CAD build for the part. Positions are in the model's coordinates, mm. A direction names the side the tool comes from. Give positions to 0.01 mm unless a question says otherwise; leave off trailing zeros. Order: outer loops, then holes, each group sorted by start corner. A loop starts at its lowest first (then second) coordinate and runs counter-clockwise, first axis right, second up. Notation, with made-up numbers: (-32.75, 29.25) -> (-28.75, 29.25) arc R13 cw to (-28.75, 40.25) -> close; hole circle Ø8 at (79, 17.5). An arc over 180 degrees is marked (long way). Use one line per item in the form item = value. Start each with the question number.
1) Cut at B-B, the plane y = -56.5. Give the cut face in (x, z), and give its area (3 significant figures).
2) Drop flat-ended pins along their axis: P1, Ø2, axis at y = -70.5, z = 0.5, coming from the +X side; P2, Ø3, axis at x = 185, y = -40, coming from the -Z side; P3, Ø4, axis at x = 15, y = -40, coming from the -Z side. Give the stop position or say it passes through.
3) Cut at A-A, the plane x = 59. Give the cut face in (y, z).
4) Mould opens along X. For faces 3 (the face through (200, -32, 2)), 4 (the face through (99, -7.833, 2)), 5 (the face through (8.555, -80.979, 2.535)), 6 (the face through (160, -42, 2)) say: pulls with the +X half, pulls with the -X half, needs draft (parallel to the pull), parting line crosses it, or undercut.
5) Probe line 1 (Y direction, x = 67, z = 4); line 2 (X direction, y = -16, z = 3.25); line 3 (Y direction, x = 185, z = 1.8). List the from-to ranges inside material, lowest first.
6) Tool access for faces 1 (the face through (40, -42, 2)), 2 (the face through (99, -7, 0)): list every direction of +Z, -Z, +X, -X, +Y, -Y with a clear straight run to the whole face (end or side of a thin tool).
7) Cut at C-C, the plane z = 1.65. State how many separate pieces and enclosed holes the cut face has, and give its area (3 significant figures).
8) Cut at D-D, the plane y = -80. Give the cut face in (x, z), and give its area (3 significant figures).
from build123d import *

# Parameters (mm, degrees)
SKETCH_W    = 200
SKETCH_H    = 87.167173
SKETCH_R    = 1.5625
SKETCH_W_2  = 120
SKETCH_H_2  = 67.742155
PAD_DEPTH   = 5
FILLET_R    = 30
FILLET001_R = 3.125
FILLET002_R = 1


with BuildPart() as part:
    # Sketch → Pad (new body)
    with BuildSketch(Plane.XY):
        with Locations((100, -46.416413)):
            Rectangle(SKETCH_W, SKETCH_H)
        with Locations((175, -10)):
            Circle(SKETCH_R, mode=Mode.SUBTRACT)
        with Locations((175, -30)):
            Circle(SKETCH_R, mode=Mode.SUBTRACT)
        with Locations((185, -20)):
            Circle(SKETCH_R, mode=Mode.SUBTRACT)
        with Locations((185, -40)):
            Circle(SKETCH_R, mode=Mode.SUBTRACT)
        with Locations((25, -10)):
            Circle(SKETCH_R, mode=Mode.SUBTRACT)
        with Locations((25, -30)):
            Circle(SKETCH_R, mode=Mode.SUBTRACT)
        with Locations((15, -20)):
            Circle(SKETCH_R, mode=Mode.SUBTRACT)
        with Locations((15, -40)):
            Circle(SKETCH_R, mode=Mode.SUBTRACT)
        with Locations((100, -41.703904)):
            Rectangle(SKETCH_W_2, SKETCH_H_2, mode=Mode.SUBTRACT)
    extrude(amount=PAD_DEPTH)

    # Fillet
    fillet_edges = [part.edges().sort_by_distance(p)[0] for p in [
        (200, -90, 2.5),
        (0, -90, 2.5),
    ]]
    fillet(fillet_edges, radius=FILLET_R)

    # Fillet001
    fillet001_edges = [part.edges().sort_by_distance(p)[0] for p in [
        (40, -7.832827, 2.5),
        (160, -7.832827, 2.5),
        (160, -75.574982, 2.5),
        (40, -75.574982, 2.5),
    ]]
    fillet(fillet001_edges, radius=FILLET001_R)

    # Fillet002
    fillet002_edges = [part.edges().sort_by_distance(p)[0] for p in [
        (0, -2.832827, 2.5),
        (200, -2.832827, 2.5),
    ]]
    fillet(fillet002_edges, radius=FILLET002_R)


solid = part.part
Result:
q1.outline = (0, 0) -> (40, 0) -> (40, 5) -> (0, 5) -> close; (160, 0) -> (200, 0) -> (200, 5) -> (160, 5) -> close
q1.area = 400 mm²
q2.P1 = 198.46
q2.P2 = through
q2.P3 = 0
q3.outline = (-90, 0) -> (-75.57, 0) -> (-75.57, 5) -> (-90, 5) -> close; (-7.83, 0) -> (-2.83, 0) -> (-2.83, 5) -> (-7.83, 5) -> close
q4.face_3 = pulls with the +X half
q4.face_4 = undercut
q4.face_5 = pulls with the -X half
q4.face_6 = undercut
q5.line_1 = -90 to -75.57, -7.83 to -2.83
q5.line_2 = 0 to 40, 160 to 200
q5.line_3 = -85.98 to -41.56, -38.44 to -21.56, -18.44 to -2.83
q6.face_1 = +Z, -Z
q6.face_2 = -Z, +X, -X, +Y, -Y
q7.separate_pieces = 1
q7.enclosed_holes = 9
q7.area = 8,860 mm²
q8.outline = (7.64, 0) -> (192.36, 0) -> (192.36, 5) -> (7.64, 5) -> close
q8.area = 924 mm²
